Part print with two shaded views. Sizes in mm from the minimum x, y, z corner. A direction names the side the tool comes from. Coordinates: 2 decimals unless noted, no trailing zeros. Order: outer loops, then holes, each group sorted by start corner. A loop starts at its lowest first (then second) coordinate and runs counter-clockwise, first axis right, second up. Notation, with made-up numbers: (-40, 84) - (18, 84) arc R11 cw to (18, 99) - close; hole circle Ø9 at (37, 80). An arc over 180 degrees is marked (long way). Return JSON: item names as keys, results as strings.
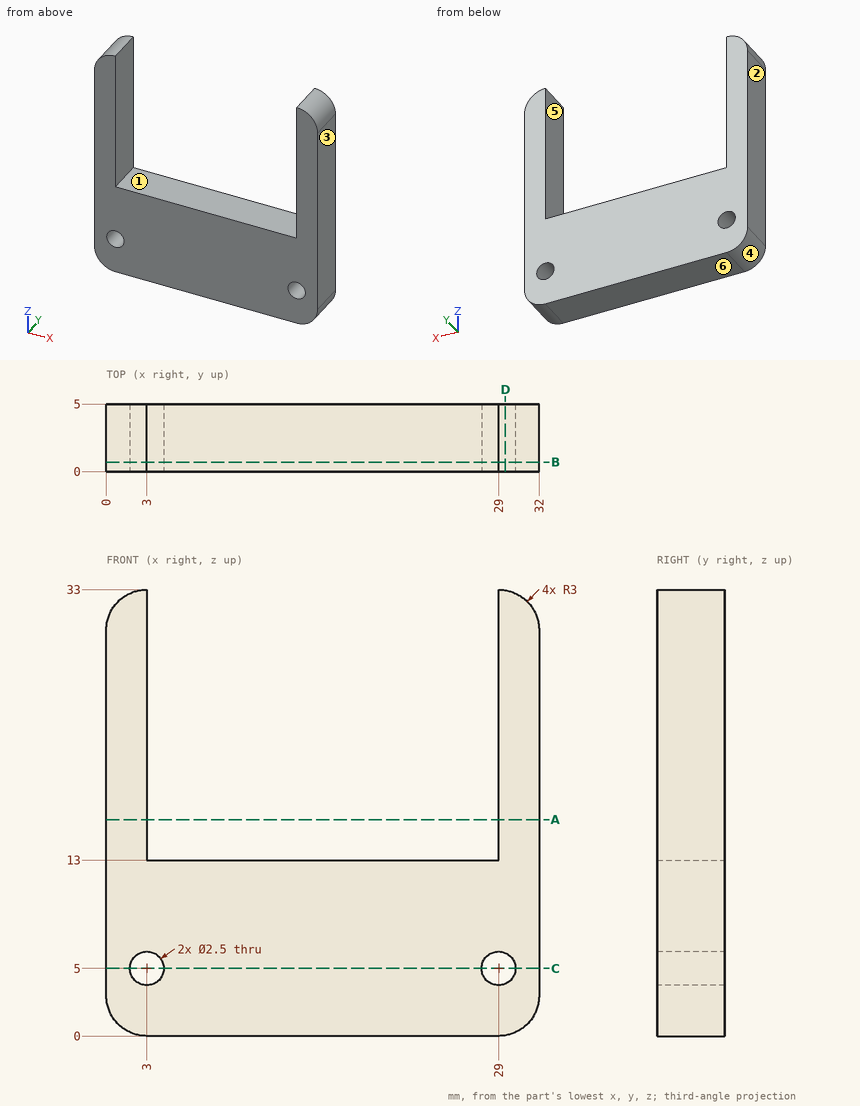
Item 1: Band-saw the part on A-A, the plane z = 16. List the corners of the cut face in (x, y), then the cut area to 3 significant figures.
Findings below:
{"outline": "(0, 0) - (3, 0) - (3, 5) - (0, 5) - close; (29, 0) - (32, 0) - (32, 5) - (29, 5) - close", "area": "30.0 mm²"}
Item 2: Drop a flat-ended pin along its axis: P1, Ø1, axis at x = 11, y = 4, coming from the +Z side. Give the stop position or say it passes through.
Findings below:
{"P1": "stops at z = 13"}
Item 3: Band-saw the part on B-B, the plane y = 0.7. Count the separate pieces of the cut face and the enclosed holes in it, then the cut area to 3 significant figures.
Findings below:
{"separate pieces": "1", "enclosed holes": "2", "area": "518 mm²"}
Item 4: Wall check: L1, parallel to X at y = 3.85, z = 5; L2, parallel to X at y = 1.2, z = 5.5; L3, parallel to X at y = 4.75, z = 24. Give the ranges that are in metal, low to high. Write a range as [from, to].
Findings below:
{"L1": "x = [0, 1.75], [4.25, 27.75], [30.25, 32]", "L2": "x = [0, 1.85], [4.15, 27.85], [30.15, 32]", "L3": "x = [0, 3], [29, 32]"}
Item 5: Which spindle directions (+Z, -Z, +X, -X, +Y, -Y) get a long thin tool onto all of the face, cutting with end or side? Do the marked faces 1 and 2. Say none if no direction does.
Findings below:
{"face 1": "+Z, +Y, -Y", "face 2": "+Z, -Z, -X, +Y, -Y"}
Item 6: Band-saw the part on D-D, the plane x = 29.5. List the corners of the cut face in (y, z), then the cut area to 3 significant figures.
Findings below:
{"outline": "(0, 0.04) - (5, 0.04) - (5, 3.85) - (0, 3.85) - close; (0, 6.15) - (5, 6.15) - (5, 32.96) - (0, 32.96) - close", "area": "153 mm²"}
Item 7: Band-saw the part on C-C, the plane z = 5. List the corners of the cut face in (x, y).
Findings below:
{"outline": "(0, 0) - (1.75, 0) - (1.75, 5) - (0, 5) - close; (4.25, 0) - (27.75, 0) - (27.75, 5) - (4.25, 5) - close; (30.25, 0) - (32, 0) - (32, 5) - (30.25, 5) - close"}
Item 8: Mould opens along X. For the marked faces 3, 4, 5 and 6 say: released by +X, released by -X, zero draft, split by the parting line, or undercut.
Findings below:
{"face 3": "released by +X", "face 4": "released by -X", "face 5": "undercut", "face 6": "zero draft"}
